from build123d import *

# Parameters (mm, degrees)
SKETCH1_W               = 25.4
SKETCH1_H               = 25.4
BOSS_EXTRUDE1_DEPTH     = 25.4
CUT_EXTRUDE1_DEPTH      = 25.4
CUT_EXTRUDE2_DEPTH      = 39.1
CUT_EXTRUDE2_DEPTH_BACK = 22.225
SKETCH4_R               = 2.7813
CUT_EXTRUDE3_DEPTH      = 22.225
SKETCH5_R               = 2.7813
CUT_EXTRUDE4_DEPTH      = 22.225


with BuildPart() as part:
    # Sketch1 → Boss-Extrude1 (new body)
    with BuildSketch(Plane(origin=(0, 0, 0), x_dir=(1, 0, 0), z_dir=(0, 1, 0))):
        Rectangle(SKETCH1_W, SKETCH1_H)
    extrude(amount=BOSS_EXTRUDE1_DEPTH)

    # Sketch2 → Cut-Extrude1 (cut)
    with BuildSketch(Plane(origin=(12.7, 0, 0), x_dir=(0, 0, -1), z_dir=(1, 0, 0))):
        Polygon((-12.7, 25.4), (12.7, 25.4), (-12.7, 0), align=None)
    extrude(amount=-CUT_EXTRUDE1_DEPTH, mode=Mode.SUBTRACT)

    # Sketch3 → Cut-Extrude2 (cut, two sides: drawn at the far end of the back side and taken through both)
    with BuildSketch(Plane(origin=(12.7, 0, 0), x_dir=(0, 0, -1), z_dir=(1, 0, 0)).offset(-CUT_EXTRUDE2_DEPTH_BACK)):
        Polygon((-82.386792847, 3.175), (-9.525, 3.175), (9.525, 3.175), (9.525, 22.225), (9.525, 95.086792847), (-93.517135624, 198.128928471), (-185.428928471, 106.217135624), align=None)
    extrude(amount=CUT_EXTRUDE2_DEPTH + CUT_EXTRUDE2_DEPTH_BACK, mode=Mode.SUBTRACT)

    # Sketch4 → Cut-Extrude3 (cut)
    with BuildSketch(Plane.XY.offset(-9.525)):
        with Locations((4.7625, 12.7)):
            Circle(SKETCH4_R)
    extrude(amount=-CUT_EXTRUDE3_DEPTH, mode=Mode.SUBTRACT)

    # Sketch5 → Cut-Extrude4 (cut)
    with BuildSketch(Plane(origin=(0, 3.175, 0), x_dir=(1, 0, 0), z_dir=(0, 1, 0))):
        with Locations(Location((4.7625, 0, 0), (0, 0, 270))):
            Circle(SKETCH5_R)
    extrude(amount=-CUT_EXTRUDE4_DEPTH, mode=Mode.SUBTRACT)


solid = part.part
CAD build for the part. Positions are in the model's coordinates, mm. A direction names the side the tool comes from. Round coordinates to 2 decimals unless told otherwise and drop trailing zeros. Loops run counter-clockwise (first coordinate to the right, second up) from the corner with the lowest first, then second, coordinate; pieces in that order, holes last.
(1) Cut at C-C (x = 4). Give the cut face in (y, z) (3 decimals).
(2) Cut at D-D (z = -6.5). Give the cut face in (x, y) (3 decimals), plus the area to 3 significant figures.
(3) Cut at A-A (y = 12.7). Give the cut face in (x, z) (3 decimals).
(4) Which spindle directions (+Z, -Z, +X, -X, +Y, -Y) get a long thin tool onto all of the face, cutting with end or side? Do faces 4 (the flat face through (1, 3.175, 0)), 5 (the flat face through (12.7, 2, -6)). Say none if no direction does.
(5) Two-plate mould, pull along Y, no slides. Class faces 1 (the flat face through (-10.3, 12.8, -0.1)), 2 (the flat face through (1, 13, -9.525)), 3 (the cylindrical face through (4.16, 9.985, -11.09)): +Y half, -Y half, draft (parallel to the pull), parting line (faces both ways), or undercut.
(6) Drop flat-ended pins along their axis: pin 1 (15 mm diameter, centred on y = 13, z = -3, fed in from +X); pin 2 (4 mm diameter, centred on x = -4, y = 5, fed in from +Z); pin 3 (12 mm diameter, centred on x = 1, z = 0, fed in from +Y) (3 decimals); pin 4 (7 mm diameter, centred on x = 4.76, y = 12.7, fed in from +Z) (3 decimals). Give the stop position or say it passes through.
(7) Cut at B-B (z = 0). Give the cut face in (x, y) (3 decimals), plus the area to 3 significant figures.
(8) Wall check: line 1 along X through (y, z) = (1.05, 0); line 2 along Y through (x, z) = (-2.5, -9) (3 decimals); line 3 along Z through (x, y) = (8.5, 4.25) (3 decimals). Give the ranges that are in metal, low to high.
Findings below:
1. outline: (0, -12.7) - (10.025, -12.7) - (10.025, -9.525) - (3.175, -9.525) - (3.175, -2.675) - (0, -2.675) - close; (0, 2.675) - (3.175, 2.675) - (3.175, 9.525) - (0, 12.7) - close; (15.375, -12.7) - (25.4, -12.7) - (22.225, -9.525) - (15.375, -9.525) - close
2. outline: (-12.7, 0) - (12.7, 0) - (12.7, 3.175) - (-9.525, 3.175) - (-9.525, 19.2) - (-12.7, 19.2) - close
2. area: 132 mm2
3. outline: (-12.7, -12.7) - (1.981, -12.7) - (1.981, -9.525) - (-9.525, -9.525) - (-9.525, 0) - (-12.7, 0) - close; (7.544, -12.7) - (12.7, -12.7) - (12.7, -9.525) - (7.544, -9.525) - close
4. face 4: +Z, +X, +Y
4. face 5: +Z, -Z, +X, +Y, -Y
5. face 1: +Y half
5. face 2: draft
5. face 3: undercut
6. pin 1: stops at x = 12.7
6. pin 2: stops at z = 9.7
6. pin 3: stops at y = 3.175
6. pin 4: stops at z = -9.525
7. outline: (-12.7, 0) - (1.981, 0) - (1.981, 3.175) - (-9.525, 3.175) - (-9.525, 12.7) - (-12.7, 12.7) - close; (7.544, 0) - (12.7, 0) - (12.7, 3.175) - (7.544, 3.175) - close
7. area: 93.2 mm2
8. line 1: x = -12.7 to 1.98, 7.54 to 12.7
8. line 2: y = 0 to 3.175
8. line 3: z = -12.7 to -9.525
